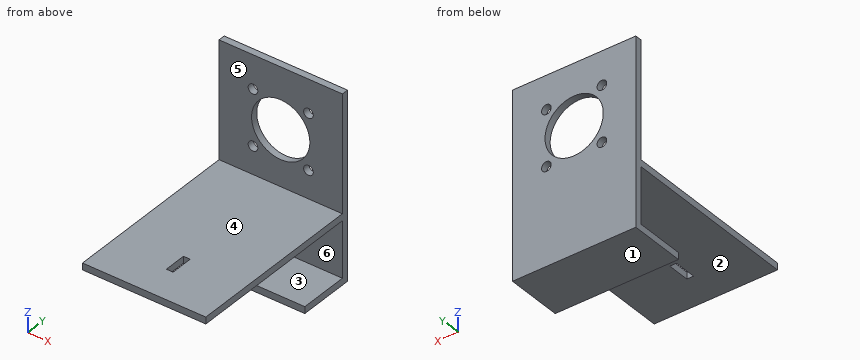
```python
from build123d import *

# Parameters (mm, degrees)
SKETCH1_W           = 55
SKETCH1_H           = 80
SKETCH1_R           = 13
SKETCH1_R_2         = 2.15
BOSS_EXTRUDE2_DEPTH = 3
SKETCH2_W           = 55
SKETCH2_H           = 3
BOSS_EXTRUDE3_DEPTH = 80
SKETCH3_W           = 3
SKETCH3_H           = 10
CUT_EXTRUDE1_DEPTH  = 80
SKETCH4_W           = 55
SKETCH4_H           = 25
BOSS_EXTRUDE4_DEPTH = 3


with BuildPart() as part:
    # Sketch1 → Boss-Extrude2 (new body)
    with BuildSketch(Plane(origin=(0, 0, 0), x_dir=(1, 0, 0), z_dir=(0, 1, 0))):
        Rectangle(SKETCH1_W, SKETCH1_H)
        with Locations((0, -12.743931666)):
            Circle(SKETCH1_R, mode=Mode.SUBTRACT)
        with Locations((12.374368671, -0.369562995)):
            Circle(SKETCH1_R_2, mode=Mode.SUBTRACT)
        with Locations((12.374368671, -25.118300337)):
            Circle(SKETCH1_R_2, mode=Mode.SUBTRACT)
        with Locations((-12.374368671, -25.118300337)):
            Circle(SKETCH1_R_2, mode=Mode.SUBTRACT)
        with Locations((-12.374368671, -0.369562995)):
            Circle(SKETCH1_R_2, mode=Mode.SUBTRACT)
    extrude(amount=BOSS_EXTRUDE2_DEPTH)

    # Sketch2 → Boss-Extrude3 (add)
    with BuildSketch(Plane.XZ):
        with Locations((0, -13.5)):
            Rectangle(SKETCH2_W, SKETCH2_H)
    extrude(amount=BOSS_EXTRUDE3_DEPTH)

    # Sketch3 → Cut-Extrude1 (cut)
    with BuildSketch(Plane(origin=(0, 0, -15), x_dir=(-1, 0, 0), z_dir=(0, 0, -1))):
        with Locations((0, -60)):
            Rectangle(SKETCH3_W, SKETCH3_H)
    extrude(amount=-CUT_EXTRUDE1_DEPTH, mode=Mode.SUBTRACT)

    # Sketch4 → Boss-Extrude4 (add)
    with BuildSketch(Plane(origin=(0, 0, -40), x_dir=(-1, 0, 0), z_dir=(0, 0, -1))):
        with Locations((0, -9.5)):
            Rectangle(SKETCH4_W, SKETCH4_H)
    extrude(amount=BOSS_EXTRUDE4_DEPTH)


solid = part.part
```
Here's how the part is built. I have some questions about the finished solid (model axes, mm). Face numbers are marked on the shaded views. A direction names the side the tool comes from. Round coordinates to 2 decimals unless told otherwise and drop trailing zeros. Write each loop counter-clockwise with the first axis right and the second up, starting at its lowest first coordinate (ties: lowest second). Pieces come first, ordered by that corner, then holes. Notation, with made-up numbers: M 89,5 L 95,5 A7 cw 95,12 Z; hole C -8,61 d1. An arc over 180 degrees is marked long. Answer as CSV lines item,"result". Start each with the question number.
1. Suppose I cut it at C-C on z = 5.5. Write out the boundary of the cut face in (x, y).
2. I'm going to push flat-ended pins straight in: pin 1 Ø4 at (x, z) = (18.5, -29) entering from -Y; pin 2 Ø3.5 at (x, z) = (7, -41) entering from -Y; pin 3 Ø8 at (x, y) = (18, -62) entering from -Z; pin 4 Ø4 at (x, z) = (-12.37, 25.12) entering from -Y. Where does each tip first touch, or does it pass through?
3. I need wall thicknesses on probe 1 along Z at (x, y) = (16, -17); probe 2 along Z at (x, y) = (0, 2); probe 3 along Y at (x, z) = (20, 11). Which ranges of each line are inside material? Lowest first, please.
4. On a 3-axis mill with a long thin cutter (end or side, diameter ignored), from which of +Z, -Z, +X, -X, +Y, -Y can I reach the whole of each face in a straight line? I mean the marked faces 1 and 2. Say none if no direction works.
5. Suppose I cut it at B-B on x = 0. Write out the boundary of the cut face in (y, z).
6. Thinking about a two-plate mould opening in Z: for the marked faces 3, 4, 5 and 6, which applies, released by +Z, released by -Z, zero draft, split by the parting line, or undercut?
7. Suppose I cut it at D-D on x = 6. Write out the boundary of the cut face in (y, z).
8. Suppose I cut it at A-A on y = -18. Write out the boundary of the cut face in (x, z), then the cut area to 3 significant figures.
Check result:
1,outline,"M -27.5,0 L -10.79,0 L -10.79,3 L -27.5,3 Z; M 10.79,0 L 27.5,0 L 27.5,3 L 10.79,3 Z"
2,pin 1,"stops at y = 0"
2,pin 2,"stops at y = -22"
2,pin 3,"stops at z = -15"
2,pin 4,"passes through"
3,probe 1,"z = -43 to -40, -15 to -12"
3,probe 2,"z = -43 to -0.26, 25.74 to 40"
3,probe 3,"y = 0 to 3"
4,face 1,"-Z, +X, -X, +Y, -Y"
4,face 2,"+X, -X, -Y"
5,outline,"M -80,-15 L -65,-15 L -65,-12 L -80,-12 Z; M -55,-15 L 0,-15 L 0,-40 L -22,-40 L -22,-43 L 3,-43 L 3,-0.26 L 0,-0.26 L 0,-12 L -55,-12 Z; M 0,25.74 L 3,25.74 L 3,40 L 0,40 Z"
6,face 3,"undercut"
6,face 4,"released by +Z"
6,face 5,"zero draft"
6,face 6,"undercut"
7,outline,"M -80,-15 L 0,-15 L 0,-40 L -22,-40 L -22,-43 L 3,-43 L 3,1.21 L 0,1.21 L 0,-12 L -80,-12 Z; M 0,24.28 L 3,24.28 L 3,40 L 0,40 Z"
8,outline,"M -27.5,-43 L 27.5,-43 L 27.5,-40 L -27.5,-40 Z; M -27.5,-15 L 27.5,-15 L 27.5,-12 L -27.5,-12 Z"
8,area,"330 mm2"
